Input: part model. Units: mm. Frame: model coordinates. A direction names the side the tool comes from. Round coordinates to 2 decimals unless told otherwise and drop trailing zeros. Loops run counter-clockwise (first coordinate to the right, second up) from the corner with the lowest first, then second, coordinate; pieces in that order, holes last.
1) First-contact query: pin 1 (12 mm diameter, centred on x = -2.5, y = -24, fed in from +Z); pin 2 (6.5 mm diameter, centred on y = -9.39, z = 88.9, fed in from -X). Flat tips, straight axial feed; report the tip coordinate or a pass-through.
2) Section A-A, the plane z = 49. Return loops of the section in (x, y), and give its area (3 significant figures).
3) Ray query, line 1 along Y through (x, z) = (-2.5, 499.5); line 2 along X through (y, z) = (15, 444); line 3 along X through (y, z) = (-3, 37). Return the intervals inside material, ascending.
4) Access query for faces 1 (the face through (-11.527, -6.532, 486.215)), 2 (the face through (-10.901, -9, 275)). Directions: +Z, -Z, +X, -X, +Y, -Y. A direction counts if a zero-diameter tool reaches every point of the face in a straight line with its end or side. Return the directions, or none.
5) Draft query along X for faces 3 (the face through (12.6, -14.86, 139.2)), 4 (the face through (-12.171, -10, 275)), 5 (the face through (11.959, -10, 275)). Return one class per face: pulls with the +X half, pulls with the -X half, needs draft (parallel to the pull), parting line crosses it, or undercut.
Autodesk Inventor part; units mm, degrees
ref_plane "YZ Plane" through (0, 0, 0) normal (1, 0, 0) x (0, 1, 0)
ref_plane "XZ Plane" through (0, 0, 0) normal (0, 1, 0) x (-1, 0, 0)
ref_plane "XY Plane" through (0, 0, 0) normal (0, 0, 1) x (1, 0, 0)
sketch "Sketch1" plane through (0, 0, 0) normal (0, 0, 1) x (1, 0, 0)
  line L0 (-12.1708, 16.0073) -> (13.2292, 16.0073)
  line L1 (13.2292, 16.0073) -> (13.2292, -34.7927)
  line L2 (13.2292, -34.7927) -> (-12.1708, -34.7927)
  line L3 (-12.1708, -34.7927) -> (-12.1708, 16.0073)
  line L4 (11.9592, 14.7373) -> (-10.9008, 14.7373)
  line L5 (-10.9008, 14.7373) -> (-10.9008, -33.5227)
  line L6 (-10.9008, -33.5227) -> (11.9592, -33.5227)
  line L7 (11.9592, -33.5227) -> (11.9592, 14.7373)
  point P0 (0, 0)
  dimension "d0" = 25.4
  dimension "d1" = 50.8
  dimension "d2" = 1.27
extrude "Extrusion1" add sketch "Sketch1" along normal blind 558.8
sketch "Sketch2" plane through (-12.1708, 16.0073, 0) normal (0, 1, 0) x (1, 0, 0)
  circle A0 centre (12.7, -12.7) radius 1.7272
  line L0 (25.4, 0) -> (0, 0)
  line L1 (0, 0) -> (0, -558.8)
  point P0 (12.1708, 0)
  dimension "d5" = 3.4544
  dimension "d6" = 12.7
  dimension "d7" = 12.7
extrude "Extrusion2" cut sketch "Sketch2" against normal through all
pattern_linear "Rectangular Pattern1" count 22 spacing 25.4 along (0, 0, 1) of "Extrusion2"
sketch "Sketch4" plane through (13.2292, -34.7927, 0) normal (1, 0, 0) x (0, 0, -1)
  circle A0 centre (-406.4, 25.4) radius 14.2875
  circle A1 centre (-152.4, 25.4) radius 14.2875
  circle A2 centre (-495.3, 25.4) radius 9.525
  circle A3 centre (-63.5, 25.4) radius 9.525
  line L0 (-495.3, 25.4) -> (-63.5, 25.4) construction
  line L1 (0, 50.8) -> (-558.8, 50.8)
  line L2 (0, 0) -> (-558.8, 0)
  line L3 (-279.4, 0) -> (-279.4, 50.8) construction
  line L4 (0, 0) -> (0, 50.8)
  line L5 (-558.8, 0) -> (-558.8, 50.8)
  point P0 (0, 34.7927)
  dimension "d15" = 28.575
  dimension "d16" = 25.4
  dimension "d17" = 254
  dimension "d18" = 279.4
  dimension "d19" = 127
  dimension "d20" = 88.9
  dimension "d22" = 88.9
  dimension "d23" = 19.05
  dimension "d24" = 558.8
extrude "Extrusion3" cut sketch "Sketch4" against normal through all contours A0 | A1 | A2 | A3
sketch "Sketch5" plane through (13.2292, -34.7927, 0) normal (1, 0, 0) x (0, 0, -1)
  circle A0 centre (-495.3, 25.4) radius 9.525
  circle A1 centre (-63.5, 25.4) radius 9.525
  circle A2 centre (-495.3, 25.4) radius 25.4 construction
  circle A3 centre (-63.5, 25.4) radius 25.4 construction
  circle A4 centre (-495.3, 25.4) radius 9.525
  line L0 (-495.3, 25.4) -> (-63.5, 25.4) construction
  circle A5 centre (-469.9, 25.4) radius 2.5797
  circle A6 centre (-520.7, 25.4) radius 2.5797
  circle A7 centre (-88.9, 25.4) radius 2.5797
  circle A8 centre (-38.1, 25.4) radius 2.5797
  point P0 (0, 34.7927)
  dimension "d27" = 50.8
  dimension "d28" = 5.1594
extrude "Extrusion4" cut sketch "Sketch5" against normal through all contours A5 | A6 | A7 | A8
equation "\"d3\" = d13"
equation "\"d13\" = 558.8"
properties part number "VerseFrame 22in for Ball Suck"
Final values:
1. pin 1: passes through
1. pin 2: stops at x = -12.17
2. outline: (-12.17, -34.79) - (13.23, -34.79) - (13.23, 16.01) - (-12.17, 16.01) - close; hole (-10.9, -33.52) - (11.96, -33.52) - (11.96, 14.74) - (-10.9, 14.74) - close
2. area: 187 mm2
3. line 1: y = -34.79 to -33.52, 14.74 to 16.01
3. line 2: x = -12.17 to -1.12, 2.18 to 13.23
3. line 3: x = -12.17 to -10.9, 11.96 to 13.23
4. face 1: +X, -X
4. face 2: +Z, -Z
5. face 3: needs draft
5. face 4: pulls with the -X half
5. face 5: undercut
